Design review of the part shown in the three views and the two pictorial views. Dimensions are in mm from the part's minimum x, y and z. Round coordinates to 2 decimals unless told otherwise and drop trailing zeros. Write each loop counter-clockwise with the first axis right and the second up, starting at its lowest first coordinate (ties: lowest second). Pieces come first, ordered by that corner, then holes. Notation, with made-up numbers: (36.25, 56.5) -> (64.25, 56.5) arc R10 cw to (64.25, 61.5) -> close; hole circle Ø9 at (80.25, -25). An arc over 180 degrees is marked (long way). Answer as a JSON object with one key per item and string values. Group by question number.
1) To check wall thickness, follow probe 1 along X at (y, z) = (159, 125); probe 2 along Y at (x, z) = (201.5, 92). State the ranges of each line that lie inside material, in increasing order. Write a range as [from, to].
2) We need section B-B, the plane z = 290. Write out the cut boundary in (x, y), then the cut area to 3 significant figures.
3) We need section C-C, the plane y = 35. Write out the cut boundary in (x, z), then the cut area to 3 significant figures.
4) We need section D-D, the plane x = 353. Write out the cut boundary in (y, z).
5) Insertion check: pin 1 Ø16 at (x, z) = (635, 372) entering from +Y; pin 2 Ø22 at (y, z) = (8, 318) entering from -X; pin 3 Ø16 at (y, z) = (13.5, 525) entering from -X. Each pin has a flat end and moves straight along its axis. Give the tip position at first contact, or say it passes through.
6) We need section A-A, the plane y = 404.5. Write out the cut boundary in (x, z).
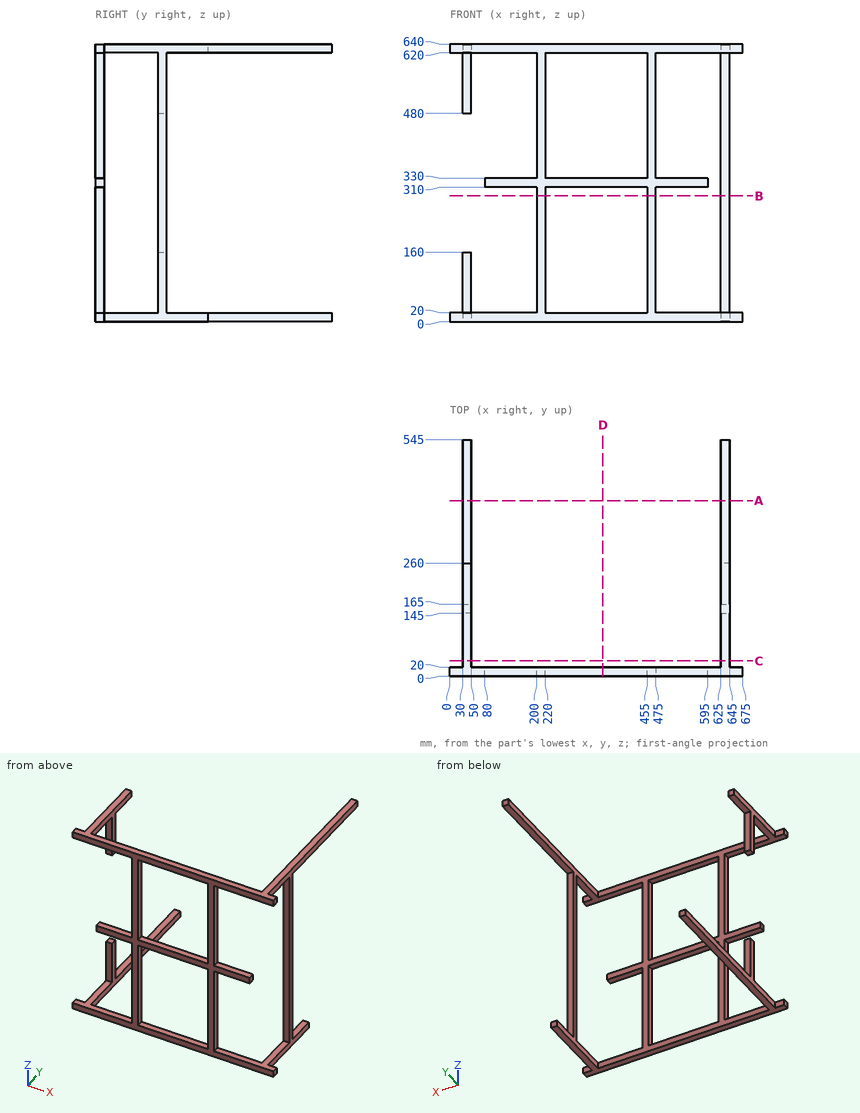
Here are the results:
{
 "1": {"probe 1": "x = [30, 50], [625, 645]", "probe 2": "y = [0, 20]"},
 "2": {"outline": "(200, 0) -> (220, 0) -> (220, 20) -> (200, 20) -> close; (455, 0) -> (475, 0) -> (475, 20) -> (455, 20) -> close; (625, 145) -> (645, 145) -> (645, 165) -> (625, 165) -> close", "area": "1,200 mm^2"},
 "3": {"outline": "(30, 0) -> (50, 0) -> (50, 20) -> (30, 20) -> close; (30, 620) -> (50, 620) -> (50, 640) -> (30, 640) -> close; (625, 0) -> (645, 0) -> (645, 20) -> (625, 20) -> close; (625, 620) -> (645, 620) -> (645, 640) -> (625, 640) -> close", "area": "1,600 mm^2"},
 "4": {"outline": "(0, 0) -> (20, 0) -> (20, 20) -> (0, 20) -> close; (0, 310) -> (20, 310) -> (20, 330) -> (0, 330) -> close; (0, 620) -> (20, 620) -> (20, 640) -> (0, 640) -> close"},
 "5": {"pin 1": "stops at y = 165", "pin 2": "stops at x = 80", "pin 3": "stops at x = 200"},
 "6": {"outline": "(30, 0) -> (50, 0) -> (50, 20) -> (30, 20) -> close; (625, 620) -> (645, 620) -> (645, 640) -> (625, 640) -> close"}
}
